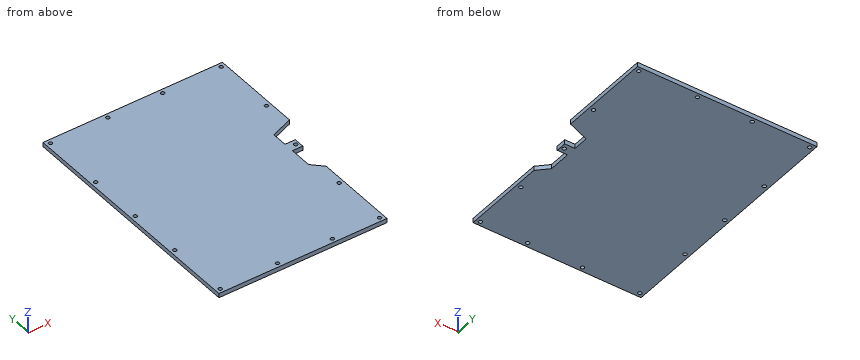
```python
from build123d import *

# Parameters (mm, degrees)
SKETCH1_R      = 0.85
EXTRUDE1_DEPTH = 2


with BuildPart() as part:
    # Sketch1 → Extrude1 (new body)
    with BuildSketch(Plane.XY):
        Polygon((-79.375, -56.4375), (-79.375, 56.4375), (3.675, 56.4375), (3.675, 13.405219977), (-6.35, 9.525), (-6.35, 2.4), (-1.5875, 2.4), (-1.5875, -2.4), (-6.35, -2.4), (-6.35, -12.7), (-1.5875, -17.4625), (-1.5875, -56.4375), align=None)
        with Locations((-3.175, 0)):
            Circle(SKETCH1_R, mode=Mode.SUBTRACT)
        with Locations((1.675, 54.4375)):
            Circle(SKETCH1_R, mode=Mode.SUBTRACT)
        with Locations((-25.443833121, 54.4375)):
            Circle(SKETCH1_R, mode=Mode.SUBTRACT)
        with Locations((-50.829063022, 54.4375)):
            Circle(SKETCH1_R, mode=Mode.SUBTRACT)
        with Locations((-77.375, 54.4375)):
            Circle(SKETCH1_R, mode=Mode.SUBTRACT)
        with Locations((-77.375, 25.386437646)):
            Circle(SKETCH1_R, mode=Mode.SUBTRACT)
        with Locations((-77.375, 0)):
            Circle(SKETCH1_R, mode=Mode.SUBTRACT)
        with Locations((-77.375, -25.408441217)):
            Circle(SKETCH1_R, mode=Mode.SUBTRACT)
        with Locations((-77.375, -54.4375)):
            Circle(SKETCH1_R, mode=Mode.SUBTRACT)
        with Locations((-50.829063022, -54.4375)):
            Circle(SKETCH1_R, mode=Mode.SUBTRACT)
        with Locations((-25.443833121, -54.4375)):
            Circle(SKETCH1_R, mode=Mode.SUBTRACT)
        with Locations((-3.5875, -54.4375)):
            Circle(SKETCH1_R, mode=Mode.SUBTRACT)
        with Locations((-3.5875, -28.51830741)):
            Circle(SKETCH1_R, mode=Mode.SUBTRACT)
        with Locations((1.675, 25.386437646)):
            Circle(SKETCH1_R, mode=Mode.SUBTRACT)
    extrude(amount=EXTRUDE1_DEPTH)


solid = part.part
```
Input: part model. Units: mm. Frame: model coordinates. Round coordinates to 2 decimals unless told otherwise and drop trailing zeros. Loops run counter-clockwise (first coordinate to the right, second up) from the corner with the lowest first, then second, coordinate; pieces in that order, holes last. Notation, with made-up numbers: (-22, 45) -> (2, 45) arc R9 cw to (2, 49) -> close; hole circle Ø2 at (59, -8.75). An arc over 180 degrees is marked (long way). Use one line per item in the form item = value. Start each with the question number.
Item 1: Section query A-A on y = -5.5. Return the cut outline in (x, z) (3 decimals), then the cut area to 3 significant figures.
Item 2: Contact query for a flat-ended pin moving along its axis: pin 1 Ø0.6 at (y, z) = (-9, 1.5) entering from +X. Output: stop coordinate, or through.
Item 3: Section query B-B on z = 0.3. Count the separate pieces of the cut face and the enclosed holes in it, then the cut area to 3 significant figures.
Item 4: Material intervals for L1, parallel to Y at x = -5, z = 1.2; L2, parallel to X at y = -34.5, z = 0.6 (1 decimal); L3, parallel to X at y = 5, z = 1.7 (3 decimals), sorted ascending. Write a range as from..to.
Item 5: Section query C-C on y = -32. Return the cut outline in (x, z) (1 decimal), then the cut area to 3 significant figures.
Ans:
q1.outline = (-79.375, 0) -> (-6.35, 0) -> (-6.35, 2) -> (-79.375, 2) -> close
q1.area = 146 mm^2
q2.pin_1 = -6.35
q3.separate_pieces = 1
q3.enclosed_holes = 14
q3.area = 8,880 mm^2
q4.L1 = -56.44..-14.05, -2.4..2.4, 10.05..56.44
q4.L2 = -79.4..-1.6
q4.L3 = -79.375..-6.35
q5.outline = (-79.4, 0) -> (-1.6, 0) -> (-1.6, 2) -> (-79.4, 2) -> close
q5.area = 156 mm^2
